Work out the finished part from the listing and answer in its coordinate system (mm). Round coordinates to 2 decimals unless told otherwise and drop trailing zeros. Write each loop counter-clockwise with the first axis right and the second up, starting at its lowest first coordinate (ties: lowest second). Pieces come first, ordered by that corner, then holes. Notation, with made-up numbers: M 56,-25.5 L 97,-25.5 A33 cw 97,5.5 Z; hole C 87.5,42 d1. An arc over 180 degrees is marked long. Answer in a Markdown table with one row per item.
```python
from build123d import *

# Parameters (mm, degrees)
SKETCH58_R          = 3.2639
BOSS_EXTRUDE1_DEPTH = 0.79375


with BuildPart() as part:
    # Sketch58 → Boss-Extrude1 (new, symmetric)
    with BuildSketch(Plane.XY.offset(-139.7)):
        with BuildLine():
            Line((-65.080499238, 1085.818309343), (-54.72678345, 1081.782441948))
            ThreePointArc((-54.72678345, 1081.782441948), (-51.218723763, 1078.418829178), (-51.116584369, 1073.559822986))
            Line((-51.116584369, 1073.559822986), (-58.03521419, 1055.810595921))
            ThreePointArc((-58.03521419, 1055.810595921), (-61.398826959, 1052.302536234), (-66.257833152, 1052.20039684))
            Line((-66.257833152, 1052.20039684), (-76.611548939, 1056.236264235))
            Line((-76.611548939, 1056.236264235), (-65.080499238, 1085.818309343))
        make_face()
        with Locations((-57.03299339, 1075.866032926)):
            Circle(SKETCH58_R, mode=Mode.SUBTRACT)
        with Locations((-63.951623211, 1058.116805861)):
            Circle(SKETCH58_R, mode=Mode.SUBTRACT)
    extrude(amount=BOSS_EXTRUDE1_DEPTH, both=True)


solid = part.part
```
1. The part is cut by section B-B (z = -139.4). Determine the outline of the cut face in (x, y).
Calculated:
| item | result |
|---|---|
| outline | M -76.61,1056.24 L -66.26,1052.2 A6.35 ccw -58.04,1055.81 L -51.12,1073.56 A6.35 ccw -54.73,1081.78 L -65.08,1085.82 Z; hole C -63.95,1058.12 d6.53; hole C -57.03,1075.87 d6.53 |
2. The part is cut by section C-C (y = 1074.5). Determine the outline of the cut face in (x, z), plus the area to 3 significant figures.
Calculated:
| item | result |
|---|---|
| outline | M -69.49,-140.49 L -60,-140.49 L -60,-138.91 L -69.49,-138.91 Z; M -54.07,-140.49 L -50.83,-140.49 L -50.83,-138.91 L -54.07,-138.91 Z |
| area | 20.2 mm² |
3. Determine the mould class of faces 1 (the flat face through (-71.36, 1054.19, -139.69)), 2 (the cylindrical face through (-64.377, 1061.353, -139.711)), 3 (the flat face through (-59.98, 1083.83, -139.69)) for opening direction Y: released by +Y, released by -Y, zero draft, split by the parting line, or undercut.
Calculated:
| item | result |
|---|---|
| face 1 | released by -Y |
| face 2 | undercut |
| face 3 | released by +Y |
4. The part is cut by section A-A (y = 1059.5). Determine the outline of the cut face in (x, z).
Calculated:
| item | result |
|---|---|
| outline | M -75.34,-140.49 L -66.91,-140.49 L -66.91,-138.91 L -75.34,-138.91 Z; M -61,-140.49 L -56.6,-140.49 L -56.6,-138.91 L -61,-138.91 Z |
5. Consider line 1 along Y through (x, z) = (-64, -139.55); line 2 along Y through (x, z) = (-61, -140.1); line 3 along X through (y, z) = (1073, -139.85). Determine where each line is inside the solid, lowest interval first. Write a range as from..to.
Calculated:
| item | result |
|---|---|
| line 1 | y = 1051.77..1054.85, 1061.38..1085.4 |
| line 2 | y = 1052.49..1056.72, 1059.51..1084.23 |
| line 3 | x = -70.08..-58.59, -55.47..-51.33 |
6. The part is cut by section D-D (x = -70.25). Determine the outline of the cut face in (y, z), plus the area to 3 significant figures.
Calculated:
| item | result |
|---|---|
| outline | M 1053.76,-140.49 L 1072.56,-140.49 L 1072.56,-138.91 L 1053.76,-138.91 Z |
| area | 29.8 mm² |
